```python
from build123d import *

# Parameters (mm, degrees)
F0_W     = 1219.2
F0_H     = 38.1
F1_DEPTH = 50.8
F2_W     = 38.1
F2_H     = 25.4
F3_DEPTH = 38.1


with BuildPart() as f1:
    # F0 (on Top) → F1 (new body)
    with BuildSketch(Plane.XY):
        Rectangle(F0_W, F0_H)
    extrude(amount=F1_DEPTH)

    # F2 (on face) → F3 (cut)
    with BuildSketch(Plane.XZ.offset(19.05)):
        with Locations((590.55, 12.7)):
            Rectangle(F2_W, F2_H)
        with Locations((-590.55, 12.7)):
            Rectangle(F2_W, F2_H)
    extrude(amount=-F3_DEPTH, mode=Mode.SUBTRACT)


solid = f1.part
```
The model under review builds one solid part; all positions refer to its coordinate system, in mm. A direction names the side the tool comes from. Give positions to 0.01 mm unless a question says otherwise; leave off trailing zeros. Write each loop counter-clockwise with the first axis right and the second up, starting at its lowest first coordinate (ties: lowest second). Pieces come first, ordered by that corner, then holes. Notation, with made-up numbers: M 35.5,63.25 L 42.5,63.25 A14 cw 42.5,87.25 Z; hole C 38.5,62.5 d4. An arc over 180 degrees is marked long. Write item = value, one per line. Start each with the question number.
Q1. We need section A-A (y = 12.5). State the section outline as (x, z) points, plus the area to 3 significant figures.
Q2. For line 1 (X direction, y = 16, z = 23), list the stretches that pass through material, from the lowest coordinate up.
Q3. Clearance check with flat-ended pins moving along their axes: pin 1 (4 mm diameter, centred on x = 45.5, y = -9, fed in from -Z); pin 2 (7.5 mm diameter, centred on y = 2.5, z = 13, fed in from -X); pin 3 (19 mm diameter, centred on x = 597.5, y = 8, fed in from -Z); pin 4 (1.5 mm diameter, centred on y = 4.5, z = 14.5, fed in from +X). State where each tip first meets the part, or that it passes through.
Q4. Machinability: for faces 1 (the face through (-591, 0, 25.4)), 2 (the face through (590, 0, 25.4)), 3 (the face through (-8, 0, 0)), which of the approach directions +Z, -Z, +X, -X, +Y, -Y give a long, thin tool a straight path to every point of the face, cutting with its end or side? Answer none if there is none.
Result set:
q1.outline = M -609.6,25.4 L -571.5,25.4 L -571.5,0 L 571.5,0 L 571.5,25.4 L 609.6,25.4 L 609.6,50.8 L -609.6,50.8 Z
q1.area = 60,000 mm2
q2.line_1 = -571.5 to 571.5
q3.pin_1 = 0
q3.pin_2 = -571.5
q3.pin_3 = 25.4
q3.pin_4 = 571.5
q4.face_1 = -Z, -X, +Y, -Y
q4.face_2 = -Z, +X, +Y, -Y
q4.face_3 = -Z, +X, -X, +Y, -Y
